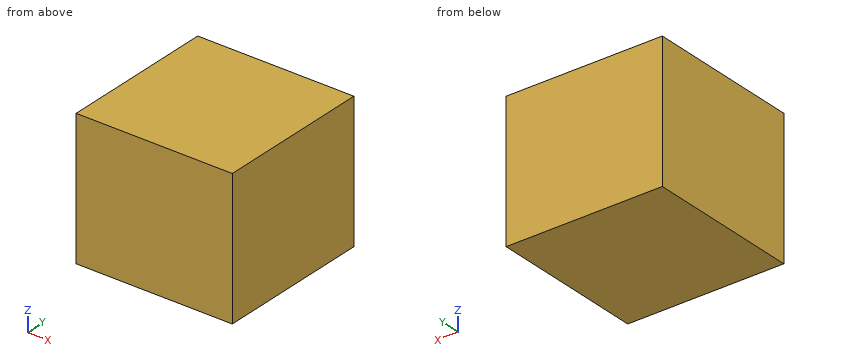
```python
from build123d import *

# Parameters (mm, degrees)
SKETCH4_W           = 40
SKETCH4_H           = 40
BOSS_EXTRUDE2_DEPTH = 35
CUT_EXTRUDE1_START  = -3
SKETCH5_W           = 34
SKETCH5_H           = 34
CUT_EXTRUDE1_DEPTH  = 29


with BuildPart() as part:
    # Sketch4 → Boss-Extrude2 (new body)
    with BuildSketch(Plane(origin=(0, 0, -10), x_dir=(-1, 0, 0), z_dir=(0, 0, -1))):
        with Locations((-105, 0)):
            Rectangle(SKETCH4_W, SKETCH4_H)
    extrude(amount=BOSS_EXTRUDE2_DEPTH)

    # Sketch5 → Cut-Extrude1 (cut)
    with BuildSketch(Plane(origin=(0, 0, -45), x_dir=(-1, 0, 0), z_dir=(0, 0, -1)).offset(CUT_EXTRUDE1_START)):
        with Locations((-105, 0)):
            Rectangle(SKETCH5_W, SKETCH5_H)
    extrude(amount=-CUT_EXTRUDE1_DEPTH, mode=Mode.SUBTRACT)


solid = part.part
```
Work out the finished part from the listing and answer in its coordinate system (mm). Coordinates: 2 decimals unless noted, no trailing zeros. Loops run counter-clockwise (first coordinate to the right, second up) from the corner with the lowest first, then second, coordinate; pieces in that order, holes last.
1) Consider probe 1 along X at (y, z) = (7, -17); probe 2 along Y at (x, z) = (106, -29); probe 3 along Z at (x, y) = (117.5, 11). Determine where each line is inside the solid, lowest interval first.
Results:
probe 1: x = 85 to 88, 122 to 125
probe 2: y = -20 to -17, 17 to 20
probe 3: z = -45 to -42, -13 to -10
2) Section A-A (x = 118) is taken. Give the vertices of the cut face in (y, z), plus the area to 3 significant figures.
Results:
outline: (-20, -45) - (20, -45) - (20, -10) - (-20, -10) - close; hole (-17, -42) - (17, -42) - (17, -13) - (-17, -13) - close
area: 414 mm2
3) Section B-B (y = -2.5) is taken. Give the vertices of the cut face in (x, z).
Results:
outline: (85, -45) - (125, -45) - (125, -10) - (85, -10) - close; hole (88, -42) - (122, -42) - (122, -13) - (88, -13) - close
